Answer from the drawing. Dimensions are ordinates in mm from the lowest x, y and z of the part. Give positions to 0.01 mm unless a question says otherwise; leave off trailing zeros. Order: outer loops, then holes, each group sorted by start corner. A loop starts at its lowest first (then second) coordinate and runs counter-clockwise, first axis right, second up. Notation, with made-up numbers: (-25.5, 22.5) - (28.5, 22.5) arc R21 ccw to (28.5, 47.5) - close; hole circle Ø11 at (-27, 40.25). An arc over 180 degrees is marked (long way). Write each question's results on one line, items separated by ' | '.
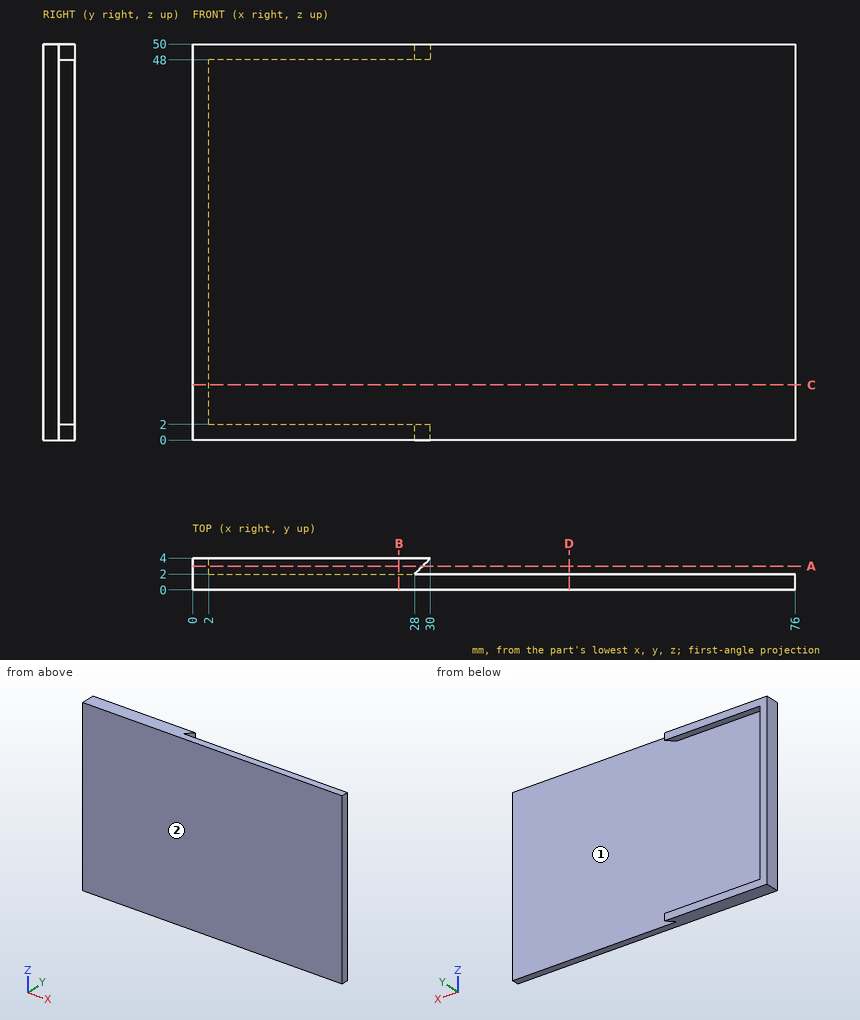
1. A cutting plane is placed at B-B, the plane x = 26. Write down the section's boundary in (y, z).
Answer list:
outline: (0, 0) - (4, 0) - (4, 2) - (2, 2) - (2, 48) - (4, 48) - (4, 50) - (0, 50) - close
2. A cutting plane is placed at A-A, the plane y = 3. Write down the section's boundary in (x, z).
Answer list:
outline: (0, 0) - (29, 0) - (29, 2) - (2, 2) - (2, 48) - (29, 48) - (29, 50) - (0, 50) - close
3. Determine the mould class of the marked faces 1 and 2 for opening direction Z: +Z half, -Z half, draft (parallel to the pull), parting line (faces both ways), or undercut.
Answer list:
face 1: undercut | face 2: draft
4. Given P1, Ø1, axis at x = 26, z = 28.5, coming from the +Y side; P2, Ø1, axis at y = 3, z = 20.5, coming from the +X side, each flat-ended and moving along its own axis, determine where each tip first touches the part or whether it passes through.
Answer list:
P1: y = 2 | P2: x = 2
5. A cutting plane is placed at C-C, the plane z = 7. Write down the section's boundary in (x, y), then the cut area to 3 significant figures.
Answer list:
outline: (0, 0) - (76, 0) - (76, 2) - (2, 2) - (2, 4) - (0, 4) - close | area: 156 mm^2
6. A cutting plane is placed at D-D, the plane x = 47.5. Write down the section's boundary in (y, z).
Answer list:
outline: (0, 0) - (2, 0) - (2, 50) - (0, 50) - close
7. Straight lines are drawn through the part: line 1 (Z direction, x = 13, y = 2.65); line 2 (Y direction, x = 31.5, z = 24.5). For each, find the intervals that lie inside material, in ascending order. Write a range as [from, to].
Answer list:
line 1: [0, 2], [48, 50] | line 2: [0, 2]
